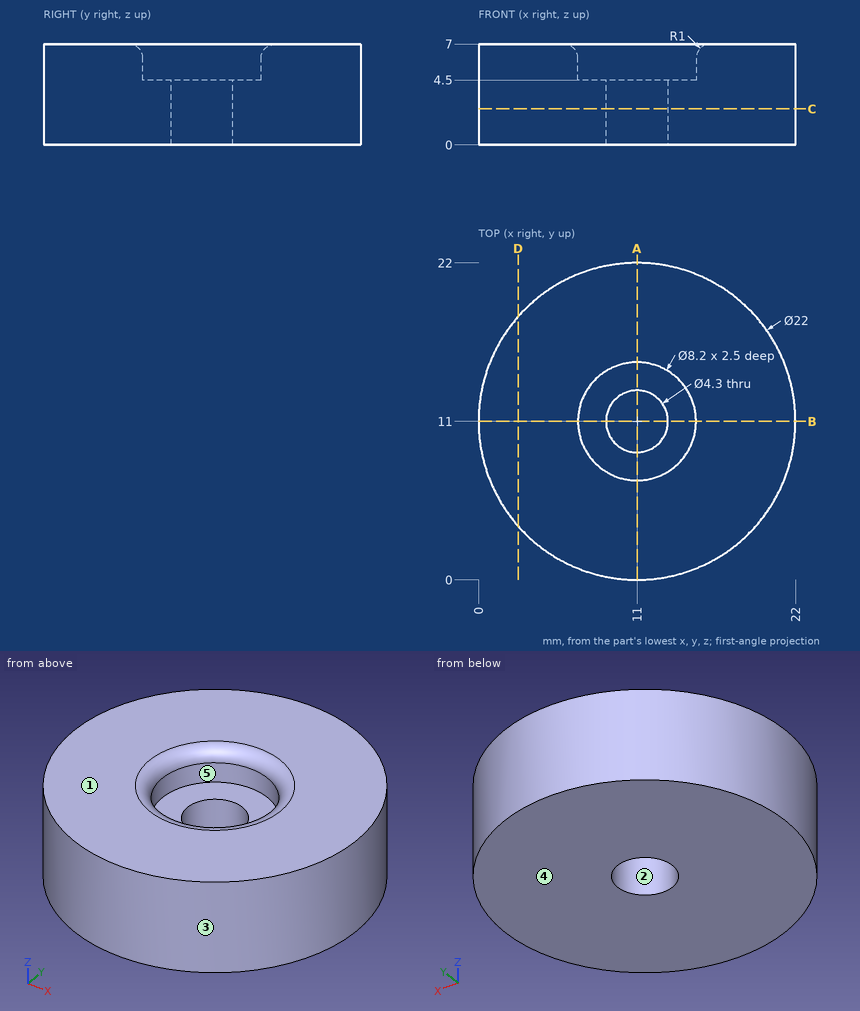
Study the drawing (mm; zero at the part's minimum x, y, z) and answer. A direction names the side the tool comes from. Give positions to 0.01 mm unless a question says otherwise; leave off trailing zeros. Order: outer loops, then holes, each group sorted by start corner. A loop starts at its lowest first (then second) coordinate and runs counter-clockwise, first axis right, second up. Notation, with made-up numbers: (74, 89) -> (103, 89) arc R33 ccw to (103, 120) -> close; hole circle Ø11 at (40, 8.25). An arc over 180 degrees is marked (long way). Put each result on its own line as item: value.
Item 1: A cutting plane is placed at A-A on x = 11. Give the vertices of the cut face in (y, z), plus the area to 3 significant figures.
Established:
outline: (0, 0) -> (8.85, 0) -> (8.85, 4.5) -> (6.9, 4.5) -> (6.9, 6) arc R1 ccw to (5.9, 7) -> (0, 7) -> close; (13.15, 0) -> (22, 0) -> (22, 7) -> (16.1, 7) arc R1 ccw to (15.1, 6) -> (15.1, 4.5) -> (13.15, 4.5) -> close
area: 114 mm^2
Item 2: For a pull along X with two mould halves and no side action, classify the marked faces 1, 2 and 3 as released by +X, released by -X, zero draft, split by the parting line, or undercut.
Established:
face 1: zero draft
face 2: undercut
face 3: split by the parting line
Item 3: For the marked faces 4 and 5, determine the directions among +Z, -Z, +X, -X, +Y, -Y from which every point of the face is accessible in a straight line to the end or side of a thin tool.
Established:
face 4: -Z, +X, -X, +Y, -Y
face 5: +Z
Item 4: Given P1, Ø1.5, axis at x = 8.5, y = 10.5, coming from the +Z side; P2, Ø7, axis at x = 11, y = 11, coming from the -Z side; P3, Ø1, axis at x = 16, z = 5.5, coming from the +Y side; P4, Ø1.5, axis at y = 15, z = 6, coming from the +X side, each flat-ended and moving along its own axis, determine where each tip first touches the part or whether it passes through.
Established:
P1: stops at z = 4.5
P2: stops at z = 0
P3: stops at y = 21.04
P4: stops at x = 21.51
Item 5: A cutting plane is placed at D-D on x = 2.75. Give the vertices of the cut face in (y, z).
Established:
outline: (3.72, 0) -> (18.28, 0) -> (18.28, 7) -> (3.72, 7) -> close
Item 6: A cutting plane is placed at C-C on z = 2.5. Give the vertices of the cut face in (x, y).
Established:
outline: circle Ø22 at (11, 11); hole circle Ø4.3 at (11, 11)
Item 7: Straight lines are drawn through the part: line 1 (Y direction, x = 11, z = 1.9); line 2 (Y direction, x = 11, z = 5.3); line 3 (X direction, y = 10.25, z = 4). For each, find the intervals that lie inside material, in ascending order.
Established:
line 1: y = 0 to 8.85, 13.15 to 22
line 2: y = 0 to 6.9, 15.1 to 22
line 3: x = 0.03 to 8.99, 13.01 to 21.97
